For this review, take the finished solid that the model builds, in its own axes (mm). Round coordinates to 2 decimals unless told otherwise and drop trailing zeros. Order: outer loops, then holes, each group sorted by start corner. A loop starts at its lowest first (then second) coordinate and runs counter-clockwise, first axis right, second up. Notation, with made-up numbers: (61.25, 51) -> (103.25, 51) arc R7 cw to (103.25, 61) -> close; hole circle Ø2 at (10, 59). An arc over 180 degrees is marked (long way). Answer in a Markdown table with one row per item.
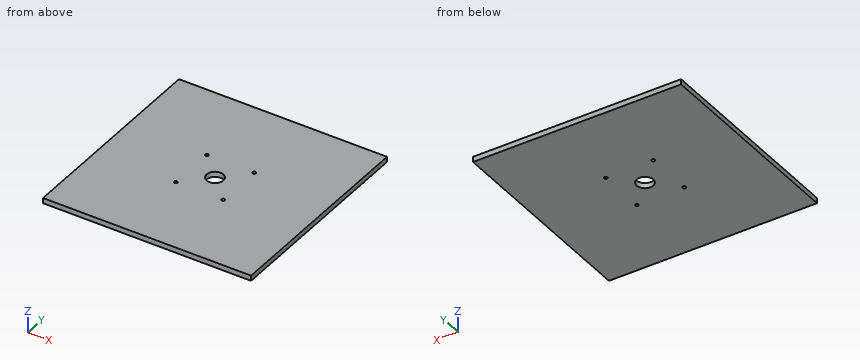
```python
from build123d import *

# Parameters (mm, degrees)
SKETCH1_W                   = 500
SKETCH1_H                   = 500
BOSS_EXTRUDE1_DEPTH         = 12.7
SKETCH4_R                   = 20
CUT_EXTRUDE1_DEPTH          = 12.7
F_8_0_MM_DOWEL_HOLES1_D     = 8
F_8_0_MM_DOWEL_HOLES1_DEPTH = 19.75
F_8_0_MM_DOWEL_HOLES1_TIP   = 2.403442476


with BuildPart() as part:
    # Sketch1 → Boss-Extrude1 (new body)
    with BuildSketch(Plane.XY):
        Rectangle(SKETCH1_W, SKETCH1_H)
    extrude(amount=BOSS_EXTRUDE1_DEPTH)

    # Sketch4 → Cut-Extrude1 (cut)
    with BuildSketch(Plane.XY.offset(12.7)):
        Circle(SKETCH4_R)
    extrude(amount=-CUT_EXTRUDE1_DEPTH, mode=Mode.SUBTRACT)

    # Ø8.0 mm Dowel Holes1
    with Locations(Plane(origin=(0, 0, 0), x_dir=(-1, 0, 0), z_dir=(0, 0, -1))):
        with Locations((57, 57), (-57, 57), (-57, -57), (57, -57)):
            Hole(F_8_0_MM_DOWEL_HOLES1_D / 2, depth=F_8_0_MM_DOWEL_HOLES1_DEPTH)
            with Locations((0, 0, -(F_8_0_MM_DOWEL_HOLES1_DEPTH + F_8_0_MM_DOWEL_HOLES1_TIP / 2))):  # 118° drill point
                Cone(0, F_8_0_MM_DOWEL_HOLES1_D / 2, F_8_0_MM_DOWEL_HOLES1_TIP, mode=Mode.SUBTRACT)


solid = part.part
```
Q1. To check wall thickness, follow probe 1 along Y at (x, z) = (-57, 8.5); probe 2 along Y at (x, z) = (0, 3.25); probe 3 along X at (y, z) = (-10.5, 10.25). State the ranges of each line that lie inside material, in increasing order.
Answer key:
| item | result |
|---|---|
| probe 1 | y = -250 to -61, -53 to 53, 61 to 250 |
| probe 2 | y = -250 to -20, 20 to 250 |
| probe 3 | x = -250 to -17.02, 17.02 to 250 |
Q2. Take a section at A-A, the plane x = 0. Write out the cut boundary in (y, z), then the cut area to 3 significant figures.
Answer key:
| item | result |
|---|---|
| outline | (-250, 0) -> (-20, 0) -> (-20, 12.7) -> (-250, 12.7) -> close; (20, 0) -> (250, 0) -> (250, 12.7) -> (20, 12.7) -> close |
| area | 5,840 mm^2 |
